For this review, take the finished solid that the model builds, in its own axes (mm). Face numbers are marked on the shaded views. Coordinates: 2 decimals unless noted, no trailing zeros. Loops run counter-clockwise (first coordinate to the right, second up) from the corner with the lowest first, then second, coordinate; pieces in that order, holes last.
1. Mouldability with a two-part tool opening along X and no side actions: class the marked faces 1 and 2 as pulls with the +X half, pulls with the -X half, needs draft (parallel to the pull), parting line crosses it, or undercut.
2. Take a section at B-B, the plane x = 35. State the section outline as (y, z) points.
3. Take a section at A-A, the plane y = 0. State the section outline as (x, z) points.
4. Clearance check with flat-ended pins moving along their axes: P1, Ø1, axis at x = 78.5, y = -3, coming from the +Z side; P2, Ø0.7, axis at y = -2.5, z = 3, coming from the +X side. State where each tip first meets the part, or that it passes through.
5. To check wall thickness, follow probe 1 along Y at (x, z) = (-87.5, 0.2); probe 2 along X at (y, z) = (5.5, 2.2); probe 3 along Z at (x, y) = (-102.5, 8). State the ranges of each line that lie inside material, in increasing order.
```python
from build123d import *

# Parameters (mm, degrees)
CROQUIS2_R              = 1.25
SALIENTE_EXTRUIR1_DEPTH = 2
CHAFL_N1_SIZE           = 1.5
SALIENTE_EXTRUIR2_DEPTH = 1
SALIENTE_EXTRUIR3_DEPTH = 0.4


with BuildPart() as part:
    # Croquis2 → Saliente-Extruir1 (new body)
    with BuildSketch(Plane.XY.offset(2)):
        with BuildLine():
            Line((-107.5, -24), (107.5, -24))
            ThreePointArc((107.5, -24), (131.5, 0), (107.5, 24))
            Line((107.5, 24), (-107.5, 24))
            ThreePointArc((-107.5, 24), (-131.5, 0), (-107.5, -24))
        make_face()
        with Locations((-87.5, -21.5)):
            Circle(CROQUIS2_R, mode=Mode.SUBTRACT)
        with Locations((-87.5, 21.5)):
            Circle(CROQUIS2_R, mode=Mode.SUBTRACT)
        with Locations((87.5, 21.5)):
            Circle(CROQUIS2_R, mode=Mode.SUBTRACT)
        with Locations((87.5, -21.5)):
            Circle(CROQUIS2_R, mode=Mode.SUBTRACT)
    extrude(amount=-SALIENTE_EXTRUIR1_DEPTH)

    # Chaflán1
    # the kernel refuses this chamfer: 1.5 mm, written as the material it takes off along each edge
    with BuildSketch(Plane(origin=(-87.5, -21.5, 2), x_dir=(1, 0, 0), z_dir=(0, -1, 0))) as chafl_n1_piece_1:
        Polygon((1.25, -CHAFL_N1_SIZE), (1.25 + CHAFL_N1_SIZE, 0), (1.25, 0), align=None)
    revolve(axis=Axis((-87.5, -21.5, 2), (0, 0, 1)), mode=Mode.SUBTRACT)
    with BuildSketch(Plane(origin=(-87.5, 21.5, 2), x_dir=(1, 0, 0), z_dir=(0, -1, 0))) as chafl_n1_piece_2:
        Polygon((1.25, -CHAFL_N1_SIZE), (1.25 + CHAFL_N1_SIZE, 0), (1.25, 0), align=None)
    revolve(axis=Axis((-87.5, 21.5, 2), (0, 0, 1)), mode=Mode.SUBTRACT)
    with BuildSketch(Plane(origin=(87.5, 21.5, 2), x_dir=(1, 0, 0), z_dir=(0, -1, 0))) as chafl_n1_piece_3:
        Polygon((1.25, -CHAFL_N1_SIZE), (1.25 + CHAFL_N1_SIZE, 0), (1.25, 0), align=None)
    revolve(axis=Axis((87.5, 21.5, 2), (0, 0, 1)), mode=Mode.SUBTRACT)
    with BuildSketch(Plane(origin=(87.5, -21.5, 2), x_dir=(1, 0, 0), z_dir=(0, -1, 0))) as chafl_n1_piece_4:
        Polygon((1.25, -CHAFL_N1_SIZE), (1.25 + CHAFL_N1_SIZE, 0), (1.25, 0), align=None)
    revolve(axis=Axis((87.5, -21.5, 2), (0, 0, 1)), mode=Mode.SUBTRACT)

    # Croquis3 → Saliente-Extruir2 (add)
    with BuildSketch(Plane.XY.offset(2)):
        with BuildLine():
            Line((-107.5, 14), (-107.5, -14))
            ThreePointArc((-107.5, -14), (-121.5, 0), (-107.5, 14))
        make_face()
        with BuildLine():
            Line((107.5, 14), (107.5, -14))
            ThreePointArc((107.5, -14), (121.5, 0), (107.5, 14))
        make_face()
    extrude(amount=SALIENTE_EXTRUIR2_DEPTH)

    # Croquis4 → Saliente-Extruir3 (add)
    # profile 1 of 2: a face of its own
    with BuildSketch(Plane.XY.offset(2)):
        with BuildLine():
            Line((-106.5, -14.966629547), (-106.5, 14.966629547))
            ThreePointArc((-106.5, 14.966629547), (-122.5, 0), (-106.5, -14.966629547))
        make_face()
        with BuildLine():
            Line((-107.5, -14), (-107.5, 14))
            ThreePointArc((-107.5, 14), (-121.5, 0), (-107.5, -14))
        make_face(mode=Mode.SUBTRACT)
    # profile 2 of 2: a face of its own
    with BuildSketch(Plane.XY.offset(2)):
        with BuildLine():
            Line((106.5, 14.966629547), (106.5, -14.966629547))
            ThreePointArc((106.5, -14.966629547), (122.5, 0), (106.5, 14.966629547))
        make_face()
        with BuildLine():
            Line((107.5, 14), (107.5, -14))
            ThreePointArc((107.5, -14), (121.5, 0), (107.5, 14))
        make_face(mode=Mode.SUBTRACT)
    extrude(amount=SALIENTE_EXTRUIR3_DEPTH)


solid = part.part
```
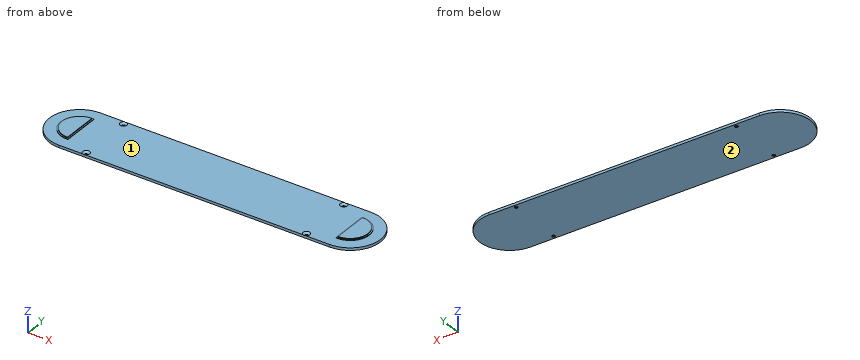
Results list:
1. face 1: undercut
1. face 2: needs draft
2. outline: (-24, 0) - (24, 0) - (24, 2) - (-24, 2) - close
3. outline: (-131.5, 0) - (131.5, 0) - (131.5, 2) - (122.5, 2) - (122.5, 2.4) - (121.5, 2.4) - (121.5, 3) - (107.5, 3) - (107.5, 2.4) - (106.5, 2.4) - (106.5, 2) - (-106.5, 2) - (-106.5, 2.4) - (-107.5, 2.4) - (-107.5, 3) - (-121.5, 3) - (-121.5, 2.4) - (-122.5, 2.4) - (-122.5, 2) - (-131.5, 2) - close
4. P1: stops at z = 2
4. P2: stops at x = 121.33
5. probe 1: y = -24 to -22.75, -20.25 to 20.25, 22.75 to 24
5. probe 2: x = -121.46 to -106.5, 106.5 to 121.46
5. probe 3: z = 0 to 2
